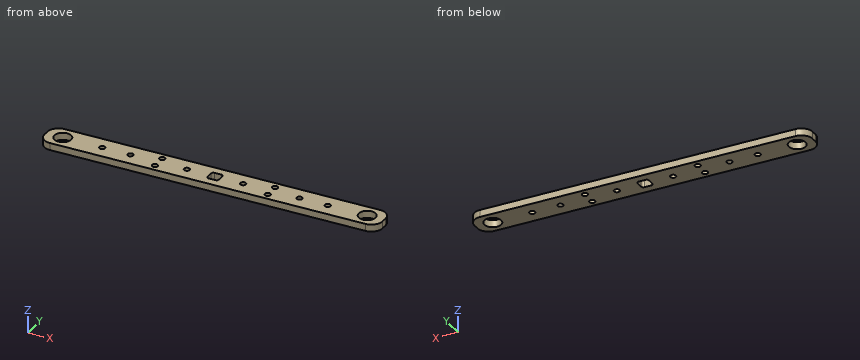
from build123d import *

# Parameters (mm, degrees)
SKETCH1_W               = 300
SKETCH1_H               = 25
SKETCH1_R               = 7.5
BOSS_EXTRUDE1_DEPTH     = 3.175
FILLET1_R               = 10
CUT_EXTRUDE1_DEPTH      = 151.653816746
CUT_EXTRUDE1_DEPTH_BACK = 151.653816746
SKETCH2_R               = 2.5
SKETCH2_W               = 10
SKETCH2_H               = 10
FILLET2_R               = 2
CUT_EXTRUDE2_DEPTH      = 151.653816746
CUT_EXTRUDE2_DEPTH_BACK = 151.653816746
SKETCH3_R               = 2.5


with BuildPart() as part:
    # Sketch1 → Boss-Extrude1 (new, symmetric)
    with BuildSketch(Plane.XY):
        Rectangle(SKETCH1_W, SKETCH1_H)
        with Locations((-135, 0)):
            Circle(SKETCH1_R, mode=Mode.SUBTRACT)
        with Locations(Location((135, 0, 0), (0, 0, 180))):
            Circle(SKETCH1_R, mode=Mode.SUBTRACT)
    extrude(amount=BOSS_EXTRUDE1_DEPTH, both=True)

    # Fillet1
    fillet1_edges = [part.edges().sort_by_distance(p)[0] for p in [
        (150, -12.5, 0),
        (-150, -12.5, 0),
        (-150, 12.5, 0),
        (150, 12.5, 0),
    ]]
    fillet(fillet1_edges, radius=FILLET1_R)

    # Sketch2 → Cut-Extrude1 (cut, two sides: drawn at the far end of the back side and taken through both)
    with BuildSketch(Plane.XY.offset(3.175).offset(-CUT_EXTRUDE1_DEPTH_BACK)):
        with Locations((-25, 0)):
            Circle(SKETCH2_R)
        with Locations((-75, 0)):
            Circle(SKETCH2_R)
        with Locations((25, 0)):
            Circle(SKETCH2_R)
        with Locations((75, 0)):
            Circle(SKETCH2_R)
        Rectangle(SKETCH2_W, SKETCH2_H)
    extrude(amount=CUT_EXTRUDE1_DEPTH + CUT_EXTRUDE1_DEPTH_BACK, mode=Mode.SUBTRACT)

    # Fillet2
    fillet2_edges = [part.edges().sort_by_distance(p)[0] for p in [
        (5, 5, 0),
        (5, -5, 0),
        (-5, -5, 0),
        (-5, 5, 0),
    ]]
    fillet(fillet2_edges, radius=FILLET2_R)

    # Sketch3 → Cut-Extrude2 (cut, two sides: drawn at the far end of the back side and taken through both)
    with BuildSketch(Plane.XY.offset(3.175).offset(-CUT_EXTRUDE2_DEPTH_BACK)):
        with Locations((-50, 6.25)):
            Circle(SKETCH3_R)
        with Locations((-50, -6.25)):
            Circle(SKETCH3_R)
        with Locations((50, -6.25)):
            Circle(SKETCH3_R)
        with Locations((50, 6.25)):
            Circle(SKETCH3_R)
        with Locations((-100, 0)):
            Circle(SKETCH3_R)
        with Locations((100, 0)):
            Circle(SKETCH3_R)
    extrude(amount=CUT_EXTRUDE2_DEPTH + CUT_EXTRUDE2_DEPTH_BACK, mode=Mode.SUBTRACT)


solid = part.part
For this review, take the finished solid that the model builds, in its own axes (mm). Give positions to 0.01 mm unless a question says otherwise; leave off trailing zeros. Loops run counter-clockwise (first coordinate to the right, second up) from the corner with the lowest first, then second, coordinate; pieces in that order, holes last. Notation, with made-up numbers: M 73,-3.75 L 98,-3.75 A23 cw 98,15.25 Z; hole C 32,85 d4. An arc over 180 degrees is marked long. Answer as a JSON object with one key per item and string values. Group by question number.
Q1. Insertion check: P1, Ø3, axis at y = -6, z = -0.5, coming from the -X side; P2, Ø4.5, axis at x = -100, y = 0, coming from the +Z side. Each pin has a flat end and moves straight along its axis. Give the tip position at first contact, or say it passes through.
Q2. Add section B-B on z = -1.75. Give the number of separate pieces and of enclosed holes in the cut face, and give its area (3 significant figures).
Q3. For probe 1 along Y at (x, z) = (50, -0.5); probe 2 along Y at (x, z) = (75, 1.75); probe 3 along Y at (x, z) = (-74.5, -0.75), list the stretches that pass through material, from the lowest coordinate up. Write a range as [from, to].
Q4. Add section A-A on x = 135. Give the boundary of the cut face in (y, z) (3 decimals).
Q5. Add section C-C on x = -50. Give the boundary of the cut face in (y, z) (3 decimals), and give its area (4 significant figures).
Checked values:
{
 "1": {"P1": "x = -149.8", "P2": "through"},
 "2": {"separate pieces": "1", "enclosed holes": "13", "area": "6,770 mm²"},
 "3": {"probe 1": "[-12.5, -8.75], [-3.75, 3.75], [8.75, 12.5]", "probe 2": "[-12.5, -2.5], [2.5, 12.5]", "probe 3": "[-12.5, -2.45], [2.45, 12.5]"},
 "4": {"outline": "M -12.5,-3.175 L -7.5,-3.175 L -7.5,3.175 L -12.5,3.175 Z; M 7.5,-3.175 L 12.5,-3.175 L 12.5,3.175 L 7.5,3.175 Z"},
 "5": {"outline": "M -12.5,-3.175 L -8.75,-3.175 L -8.75,3.175 L -12.5,3.175 Z; M -3.75,-3.175 L 3.75,-3.175 L 3.75,3.175 L -3.75,3.175 Z; M 8.75,-3.175 L 12.5,-3.175 L 12.5,3.175 L 8.75,3.175 Z", "area": "95.25 mm²"}
}
